Can you work these out from the model? Positions are in its coordinate system, mm. A direction names the side the tool comes from. Give positions to 0.01 mm unless a question says otherwise; leave off trailing zeros. Order: outer loops, then holes, each group sorted by start corner. A loop starts at its lowest first (then second) coordinate and runs counter-clockwise, first axis right, second up. Notation, with made-up numbers: (37.5, -5) - (93.5, -5) arc R28 ccw to (93.5, 28) - close; hole circle Ø5 at (60, 70). An arc over 180 degrees is marked (long way). Answer as a JSON object with one key per item and string values.
```python
from build123d import *

# Parameters (mm, degrees)
SKETCH4_W                = 25.5
SKETCH4_H                = 26
BOSS_EXTRUDE6_DEPTH      = 9.6
SKETCH17_W               = 1.117177271
SKETCH17_H               = 1.695527899
CUT_EXTRUDE3_DEPTH       = 9.6
SKETCH18_W               = 17.800407573
SKETCH18_H               = 1.75
CUT_EXTRUDE10_DEPTH      = 8
SKETCH20_W               = 16.77875935
SKETCH20_H               = 13.657573424
CUT_EXTRUDE13_DEPTH      = 10.5
SKETCH21_W               = 0.291364414
SKETCH21_H               = 1.940061713
CUT_EXTRUDE14_DEPTH      = 10.5
SKETCH22_W               = 14.860187615
SKETCH22_H               = 2.002394184
BOSS_EXTRUDE7_DEPTH      = 2
SKETCH23_W               = 7.449750672
SKETCH23_H               = 1.995003107
BOSS_EXTRUDE8_DEPTH      = 2
SKETCH24_W               = 27.5
SKETCH24_H               = 1.995003107
BOSS_EXTRUDE9_DEPTH      = 2
SKETCH25_W               = 26.3044721
SKETCH25_H               = 1.995003107
BOSS_EXTRUDE10_DEPTH     = 1.5
SKETCH19_W               = 1.2
SKETCH19_H               = 1.2
CUT_EXTRUDE15_DEPTH      = 3
CUT_EXTRUDE15_DEPTH_BACK = 18.5
SKETCH26_W               = 13.657573424
SKETCH26_H               = 1
BOSS_EXTRUDE11_DEPTH     = 1
SKETCH27_W               = 15.77875935
SKETCH27_H               = 1
BOSS_EXTRUDE12_DEPTH     = 1
SKETCH28_W               = 12.657573424
SKETCH28_H               = 1
BOSS_EXTRUDE13_DEPTH     = 1
SKETCH29_W               = 14.77875935
SKETCH29_H               = 1
BOSS_EXTRUDE14_DEPTH     = 1


with BuildPart() as part:
    # Sketch4 → Boss-Extrude6 (new body)
    with BuildSketch(Plane(origin=(-9.896990102, 0, -25.516417911), x_dir=(1, 0, 0), z_dir=(0, 1, 0))):
        with Locations((-13.336718814, -2.472262581)):
            Rectangle(SKETCH4_W, SKETCH4_H)
    extrude(amount=BOSS_EXTRUDE6_DEPTH)

    # Sketch17 → Cut-Extrude3 (cut)
    with BuildSketch(Plane(origin=(-9.896990102, 9.6, -25.516417911), x_dir=(1, 0, 0), z_dir=(0, 1, 0))):
        with Locations((-25.528130178, 9.67997347)):
            Rectangle(SKETCH17_W, SKETCH17_H)
    extrude(amount=-CUT_EXTRUDE3_DEPTH, mode=Mode.SUBTRACT)

    # Sketch18 → Cut-Extrude10 (cut)
    with BuildSketch(Plane(origin=(-9.896990102, 9.6, -25.516417911), x_dir=(1, 0, 0), z_dir=(0, 1, 0))):
        with Locations((-9.486922601, -7.147511908)):
            Rectangle(SKETCH18_W, SKETCH18_H)
    extrude(amount=-CUT_EXTRUDE10_DEPTH, mode=Mode.SUBTRACT)

    # Sketch20 → Cut-Extrude13 (cut)
    with BuildSketch(Plane(origin=(0, 9.6, -0.078786712), x_dir=(1, 0, 0), z_dir=(0, 1, 0))):
        with Locations((-20.120068773, 27.365205119)):
            Rectangle(SKETCH20_W, SKETCH20_H)
    extrude(amount=-CUT_EXTRUDE13_DEPTH, mode=Mode.SUBTRACT)

    # Sketch21 → Cut-Extrude14 (cut)
    with BuildSketch(Plane(origin=(0, 9.6, 0), x_dir=(1, 0, 0), z_dir=(0, 1, 0))):
        with Locations((-10.629391123, 35.074124474)):
            Rectangle(SKETCH21_W, SKETCH21_H)
    extrude(amount=-CUT_EXTRUDE14_DEPTH, mode=Mode.SUBTRACT)

    # Sketch22 → Boss-Extrude7 (add)
    with BuildSketch(Plane(origin=(-10.483708916, 0, 0), x_dir=(0, 0, -1), z_dir=(1, 0, 0))):
        with Locations((26.67399981, 8.598802908)):
            Rectangle(SKETCH22_W, SKETCH22_H)
    extrude(amount=BOSS_EXTRUDE7_DEPTH)

    # Sketch23 → Boss-Extrude8 (add)
    with BuildSketch(Plane(origin=(-10.483708916, 0, 0), x_dir=(0, 0, -1), z_dir=(1, 0, 0))):
        with Locations((13.769030667, 8.602498447)):
            Rectangle(SKETCH23_W, SKETCH23_H)
    extrude(amount=BOSS_EXTRUDE8_DEPTH)

    # Sketch24 → Boss-Extrude9 (add)
    with BuildSketch(Plane.XY.offset(-10.044155331)):
        with Locations((-22.233708916, 8.602498447)):
            Rectangle(SKETCH24_W, SKETCH24_H)
    extrude(amount=BOSS_EXTRUDE9_DEPTH)

    # Sketch25 → Boss-Extrude10 (add)
    with BuildSketch(Plane.ZY.offset(35.983708916)):
        with Locations((-21.196391381, 8.602498447)):
            Rectangle(SKETCH25_W, SKETCH25_H)
    extrude(amount=BOSS_EXTRUDE10_DEPTH)

    # Sketch19 → Cut-Extrude15 (cut, two sides)
    with BuildSketch(Plane(origin=(-10.483708916, 0, 0), x_dir=(0, 0, -1), z_dir=(1, 0, 0))) as cut_extrude15_sk:
        with Locations((19.843906003, 2.2)):
            Rectangle(SKETCH19_W, SKETCH19_H)
    extrude(amount=CUT_EXTRUDE15_DEPTH, mode=Mode.SUBTRACT)
    extrude(cut_extrude15_sk.sketch, amount=-CUT_EXTRUDE15_DEPTH_BACK, mode=Mode.SUBTRACT)

    # Sketch26 → Boss-Extrude11 (add)
    with BuildSketch(Plane(origin=(-28.509448448, 0, -0.078786712), x_dir=(0, 0, -1), z_dir=(1, 0, 0))):
        with Locations((27.365205119, 0.5)):
            Rectangle(SKETCH26_W, SKETCH26_H)
    extrude(amount=BOSS_EXTRUDE11_DEPTH)

    # Sketch27 → Boss-Extrude12 (add)
    with BuildSketch(Plane.XY.offset(-34.272778542)):
        with Locations((-19.620068773, 0.5)):
            Rectangle(SKETCH27_W, SKETCH27_H)
    extrude(amount=BOSS_EXTRUDE12_DEPTH)

    # Sketch28 → Boss-Extrude13 (add)
    with BuildSketch(Plane(origin=(-11.730689098, 0, -0.078786712), x_dir=(0, 0, 1), z_dir=(-1, 0, 0))):
        with Locations((-26.865205119, 0.5)):
            Rectangle(SKETCH28_W, SKETCH28_H)
    extrude(amount=BOSS_EXTRUDE13_DEPTH)

    # Sketch29 → Boss-Extrude14 (add)
    with BuildSketch(Plane(origin=(0, 0, -20.615205119), x_dir=(-1, 0, 0), z_dir=(0, 0, -1))):
        with Locations((20.120068773, 0.5)):
            Rectangle(SKETCH29_W, SKETCH29_H)
    extrude(amount=BOSS_EXTRUDE14_DEPTH)


solid = part.part
```
Q1. If we section it at B-B, the plane z = -29: Please give me the cut outline in (x, y) (3 decimals), then the cut area to 3 significant figures.
Recorded:
{"outline": "(-37.484, 7.605) - (-35.984, 7.605) - (-35.984, 0) - (-27.509, 0) - (-27.509, 1) - (-28.509, 1) - (-28.509, 9.6) - (-37.484, 9.6) - close; (-12.731, 0) - (-10.484, 0) - (-10.484, 7.598) - (-8.484, 7.598) - (-8.484, 9.6) - (-11.731, 9.6) - (-11.731, 1) - (-12.731, 1) - close", "area": "92.7 mm^2"}
Q2. I'm going to push flat-ended pins straight in: pin 1 Ø8 at (x, z) = (-19, -27.5) entering from -Y; pin 2 Ø4 at (y, z) = (1.5, -20) entering from +X; pin 3 Ø0.8 at (y, z) = (0.5, -26.5) entering from -X; pin 4 Ø1.9 at (y, z) = (4.5, -35.5) entering from -X. Where does each tip first touch, or does it pass through?
Recorded:
{"pin 1": "passes through", "pin 2": "stops at x = -10.48", "pin 3": "stops at x = -35.98", "pin 4": "stops at x = -34.87"}
Q3. If we section it at D-D, the plane z = -20: Please give me the cut outline in (x, y) (3 decimals), then the cut area to 3 significant figures.
Recorded:
{"outline": "(-37.484, 7.605) - (-35.984, 7.605) - (-35.984, 0) - (-10.484, 0) - (-10.484, 1.6) - (-28.984, 1.6) - (-28.984, 2.8) - (-10.484, 2.8) - (-10.484, 7.598) - (-8.484, 7.598) - (-8.484, 9.6) - (-37.484, 9.6) - close", "area": "230 mm^2"}
Q4. I need wall thicknesses on L1, parallel to Z at x = -27.75, y = 9; L2, parallel to Z at x = -18, y = 4.75; L3, parallel to Z at x = -14.75, y = 1.5. Which ranges of each line are inside material? Lowest first, please.
Recorded:
{"L1": "z = -36.04 to -34.27, -20.62 to -19.24, -17.49 to -8.04", "L2": "z = -36.04 to -34.27, -20.62 to -19.24, -17.49 to -10.04", "L3": "z = -36.04 to -34.27, -20.62 to -10.04"}
Q5. Which directions (+Z, -Z, +X, -X, +Y, -Y) give clear straight access to the entire face, cutting with the end or side of a thin tool? Please do faces 4 (the face through (-20, 0.5, -21.615)), 5 (the face through (-20, 2, -20.444)), 6 (the face through (-19, 6, -17.494)), 7 (the face through (-34.867, 5, -35)), 8 (the face through (-20, 5, -20.615)).
Recorded:
{"face 4": "+Y, -Y", "face 5": "+X", "face 6": "+X, +Y", "face 7": "-Z, -X, +Y, -Y", "face 8": "+Y"}
Q6. If we section it at C-C, the plane y = 6.25: Please give me the cut outline in (x, z), then the cut area to 3 significant figures.
Recorded:
{"outline": "(-35.98, -34.35) - (-34.87, -34.35) - (-34.87, -36.04) - (-10.78, -36.04) - (-10.78, -34.1) - (-10.48, -34.1) - (-10.48, -19.24) - (-28.28, -19.24) - (-28.28, -17.49) - (-10.48, -17.49) - (-10.48, -10.04) - (-35.98, -10.04) - close; hole (-28.51, -34.27) - (-11.73, -34.27) - (-11.73, -20.62) - (-28.51, -20.62) - close", "area": "400 mm^2"}
Q7. We'd pull the mould along Y, two halves only. Please class faces 1 (the face through (-20, 1, -21)), 2 (the face through (-10.484, 4, -22)), 3 (the face through (-20, 2.8, -20)): released by +Y, released by -Y, zero draft, split by the parting line, or undercut.
Recorded:
{"face 1": "released by +Y", "face 2": "zero draft", "face 3": "undercut"}
Q8. If we section it at A-A, the plane x = -18.75: Please give me the cut outline in (y, z) (3 decimals).
Recorded:
{"outline": "(0, -36.044) - (9.6, -36.044) - (9.6, -34.273) - (1, -34.273) - (1, -33.273) - (0, -33.273) - close; (0, -21.615) - (1, -21.615) - (1, -20.615) - (9.6, -20.615) - (9.6, -19.244) - (2.8, -19.244) - (2.8, -20.444) - (1.6, -20.444) - (1.6, -17.494) - (9.6, -17.494) - (9.6, -8.044) - (7.605, -8.044) - (7.605, -10.044) - (0, -10.044) - close"}
